Part model, mm, in its own coordinate system. Coordinates: 2 decimals unless noted, no trailing zeros. Write each loop counter-clockwise with the first axis right and the second up, starting at its lowest first coordinate (ties: lowest second). Pieces come first, ordered by that corner, then holes. Notation, with made-up numbers: (-31, -13) - (-4, -13) arc R27 cw to (-4, 19) - close; hole circle Ø2 at (1.25, 30.5). An arc over 180 degrees is marked (long way). Use a Markdown table: item, result.
```python
from build123d import *

# Parameters (mm, degrees)
SKETCH_1_W          = 15
SKETCH_1_H          = 15
SKETCH_1_W_2        = 12
SKETCH_1_H_2        = 12
EXTRUDE_1_DEPTH     = 300
SKETCH_2_R          = 2
CUT_EXTRUDE_1_DEPTH = 30
SKETCH_4_R          = 2.05
CUT_EXTRUDE_3_DEPTH = 120
SKETCH_5_R          = 2
CUT_EXTRUDE_4_DEPTH = 49


with BuildPart() as part:
    # 草图1 → 凸台-拉伸1 (new body)
    with BuildSketch(Plane.XY):
        Rectangle(SKETCH_1_W, SKETCH_1_H)
        Rectangle(SKETCH_1_W_2, SKETCH_1_H_2, mode=Mode.SUBTRACT)
    extrude(amount=EXTRUDE_1_DEPTH)

    # 草图2 → 切除-拉伸1 (cut)
    with BuildSketch(Plane(origin=(0, 7.5, 0), x_dir=(1, 0, 0), z_dir=(0, 1, 0))):
        with Locations(Location((0, -205, 0), (0, 0, 270))):
            Circle(SKETCH_2_R)
        with Locations(Location((0, -95, 0), (0, 0, 270))):
            Circle(SKETCH_2_R)
    extrude(amount=-CUT_EXTRUDE_1_DEPTH, mode=Mode.SUBTRACT)

    # 草图4 → 切除-拉伸3 (cut)
    with BuildSketch(Plane.ZY.offset(7.5)):
        with Locations((250, 0)):
            Circle(SKETCH_4_R)
        with Locations((260, 0)):
            Circle(SKETCH_4_R)
        with Locations(Location((40, 0, 0), (0, 0, 180))):
            Circle(SKETCH_4_R)
        with Locations(Location((50, 0, 0), (0, 0, 180))):
            Circle(SKETCH_4_R)
    extrude(amount=-CUT_EXTRUDE_3_DEPTH, mode=Mode.SUBTRACT)

    # 草图5 → 切除-拉伸4 (cut)
    with BuildSketch(Plane.ZY.offset(7.5)):
        with Locations((120, 0)):
            Circle(SKETCH_5_R)
        with Locations((110, 0)):
            Circle(SKETCH_5_R)
        with Locations(Location((190, 0, 0), (0, 0, 180))):
            Circle(SKETCH_5_R)
        with Locations(Location((180, 0, 0), (0, 0, 180))):
            Circle(SKETCH_5_R)
    extrude(amount=-CUT_EXTRUDE_4_DEPTH, mode=Mode.SUBTRACT)


solid = part.part
```
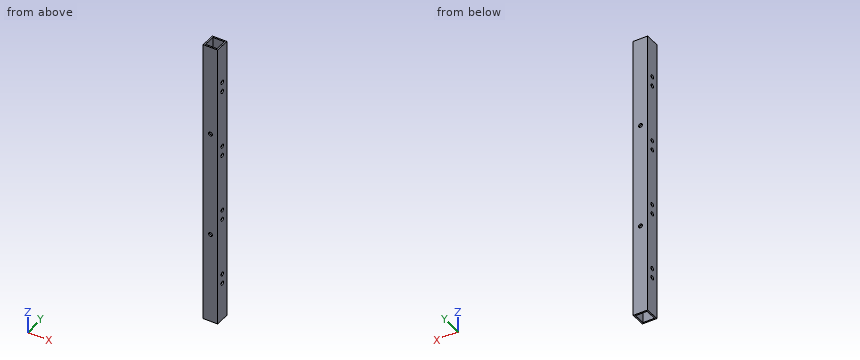
Item 1: Drill centre lines: probe 1 along Y at (x, z) = (4, 249); probe 2 along Y at (x, z) = (6.8, 120). Where is each one in solid material? Low to high.
From the geometry:
| item | result |
|---|---|
| probe 1 | -7.5 to -6, 6 to 7.5 |
| probe 2 | -7.5 to -2, 2 to 7.5 |
Item 2: Band-saw the part on A-A, the plane z = 213. Give the cut face in (x, y), then the cut area to 3 significant figures.
From the geometry:
| item | result |
|---|---|
| outline | (-7.5, -7.5) - (7.5, -7.5) - (7.5, 7.5) - (-7.5, 7.5) - close; hole (-6, -6) - (6, -6) - (6, 6) - (-6, 6) - close |
| area | 81.0 mm^2 |
Item 3: Drop a flat-ended pin along its axis: P1, Ø3, axis at y = 0, z = 120, coming from the -X side. Give the stop position or say it passes through.
From the geometry:
| item | result |
|---|---|
| P1 | through |
